The listing builds one solid part. Answer for the finished solid, in the listing's coordinates (mm). Face numbers are marked on the shaded views. A direction names the side the tool comes from. Give positions to 0.01 mm unless a question says otherwise; leave off trailing zeros. Order: outer loops, then holes, each group sorted by start corner. A loop starts at its lowest first (then second) coordinate and runs counter-clockwise, first axis right, second up. Notation, with made-up numbers: (11, 9) -> (55, 9) arc R16 cw to (55, 15) -> close; hole circle Ø5 at (25.25, 67). An arc over 180 degrees is marked (long way). Answer as a JSON object with one key per item and string values. Group by question number.
```python
from build123d import *

# Parameters (mm, degrees)
F0_R     = 13
F1_DEPTH = 36
F2_DEPTH = 12
F3_DEPTH = 25


with BuildPart() as f1:
    # F0 (on Front) → F1 (new body)
    with BuildSketch(Plane.XZ):
        with BuildLine():
            ThreePointArc((0, 19), (13.435029, 13.435029), (19, 0))
            ThreePointArc((19, 0), (13.435029, -13.435029), (0, -19))
            Line((0, -19), (40, -19))
            Line((40, -19), (40, 19))
            Line((40, 19), (0, 19))
        make_face()
        with BuildLine():
            ThreePointArc((0, -19), (-19, 0), (0, 19))
            Line((0, 19), (40, 19))
            Line((40, 19), (40, 25))
            Line((40, 25), (0, 25))
            ThreePointArc((0, 25), (-25, 0), (0, -25))
            Line((0, -25), (40, -25))
            Line((40, -25), (40, -19))
            Line((40, -19), (0, -19))
        make_face()
        with BuildLine():
            ThreePointArc((0, -19), (13.435029, -13.435029), (19, 0))
            ThreePointArc((19, 0), (13.435029, 13.435029), (0, 19))
            ThreePointArc((0, 19), (-19, 0), (0, -19))
        make_face()
        Circle(F0_R, mode=Mode.SUBTRACT)
    extrude(amount=-F1_DEPTH)

    # F0 (on Front) → F2 (cut)
    with BuildSketch(Plane.XZ):
        with BuildLine():
            ThreePointArc((0, -19), (13.435029, -13.435029), (19, 0))
            ThreePointArc((19, 0), (13.435029, 13.435029), (0, 19))
            ThreePointArc((0, 19), (-19, 0), (0, -19))
        make_face()
        Circle(F0_R, mode=Mode.SUBTRACT)
        with BuildLine():
            ThreePointArc((0, 19), (13.435029, 13.435029), (19, 0))
            ThreePointArc((19, 0), (13.435029, -13.435029), (0, -19))
            Line((0, -19), (40, -19))
            Line((40, -19), (40, 19))
            Line((40, 19), (0, 19))
        make_face()
    extrude(amount=-F2_DEPTH, mode=Mode.SUBTRACT)

    # F0 (on Front) → F3 (cut)
    with BuildSketch(Plane.XZ):
        with BuildLine():
            ThreePointArc((0, -19), (13.435029, -13.435029), (19, 0))
            ThreePointArc((19, 0), (13.435029, 13.435029), (0, 19))
            ThreePointArc((0, 19), (-19, 0), (0, -19))
        make_face()
        Circle(F0_R, mode=Mode.SUBTRACT)
    extrude(amount=-F3_DEPTH, mode=Mode.SUBTRACT)


solid = f1.part
```
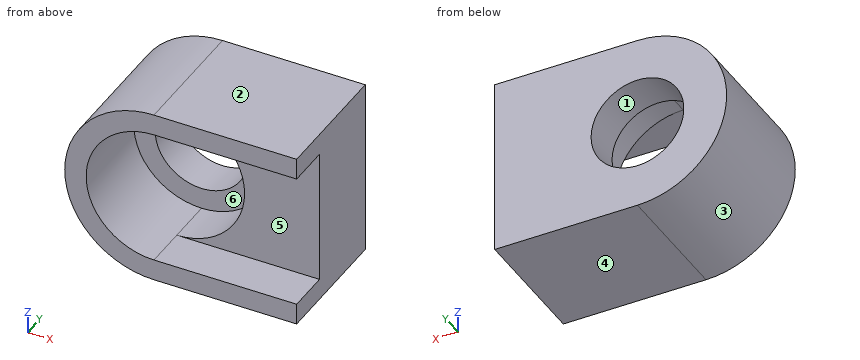
(1) Find the intervals of material crossed by line 1 along Z through (x, y) = (0, 31); line 2 along Z through (x, y) = (30.5, 11.5); line 3 along Y through (x, z) = (-15, -8.5), in increasing order. Write a range as [from, to].
(2) A cutting plane is placed at B-B (x = 24.5). Determine the outline of the cut face in (y, z), and give its area (3 significant figures).
(3) Which of the six approach directions +Z, -Z, +X, -X, +Y, -Y give full straight-line access (tool end or side, diameter ignored) to the marked faces 4, 5 and 6?
(4) A cutting plane is placed at D-D (x = 1.5). Determine the outline of the cut face in (y, z).
(5) Flat-ended cylindrical pins translate along their axes: pin 1 Ø11.5 at (x, z) = (27, 7) entering from -Y; pin 2 Ø4 at (y, z) = (6.5, -19.5) entering from -X; pin 3 Ø3 at (y, z) = (18.5, 17) entering from -X; pin 4 Ø1.5 at (x, z) = (-10, -5.5) entering from -Y. Find the tip coordinate at first contact, or state that the pin passes through.
(6) A cutting plane is placed at A-A (y = 22). Determine the outline of the cut face in (x, z), and give its area (3 significant figures).
(7) A cutting plane is placed at C-C (z = 10). Determine the outline of the cut face in (x, y).
(8) For a pull along X with two mould halves and no side action, classify the marked faces 1, 2 and 3 as +X half, -X half, draft (parallel to the pull), parting line (faces both ways), or undercut.
Check sheet entries:
{
 "1": {"line 1": "z = [-25, -13], [13, 25]", "line 2": "z = [-25, -19], [19, 25]", "line 3": "y = [25, 36]"},
 "2": {"outline": "(0, -25) -> (36, -25) -> (36, 25) -> (0, 25) -> (0, 19) -> (12, 19) -> (12, -19) -> (0, -19) -> close", "area": "1,340 mm2"},
 "3": {"face 4": "-Z, +X, -X, +Y, -Y", "face 5": "+X, -Y", "face 6": "-Y"},
 "4": {"outline": "(0, -25) -> (36, -25) -> (36, -12.91) -> (25, -12.91) -> (25, -18.94) -> (12, -18.94) -> (12, -19) -> (0, -19) -> close; (0, 19) -> (12, 19) -> (12, 18.94) -> (25, 18.94) -> (25, 12.91) -> (36, 12.91) -> (36, 25) -> (0, 25) -> close"},
 "5": {"pin 1": "stops at y = 12", "pin 2": "stops at x = -17.85", "pin 3": "stops at x = -19.62", "pin 4": "passes through"},
 "6": {"outline": "(0, -25) -> (40, -25) -> (40, 25) -> (0, 25) arc R25 ccw to start; hole (0, -19) arc R19 ccw to (19, 0) arc R19 ccw (long way) to start", "area": "1,850 mm2"},
 "7": {"outline": "(-22.91, 0) -> (-16.16, 0) -> (-16.16, 25) -> (-8.31, 25) -> (-8.31, 36) -> (-22.91, 36) -> close; (8.31, 25) -> (16.16, 25) -> (16.16, 12) -> (40, 12) -> (40, 36) -> (8.31, 36) -> close"},
 "8": {"face 1": "undercut", "face 2": "draft", "face 3": "-X half"}
}
